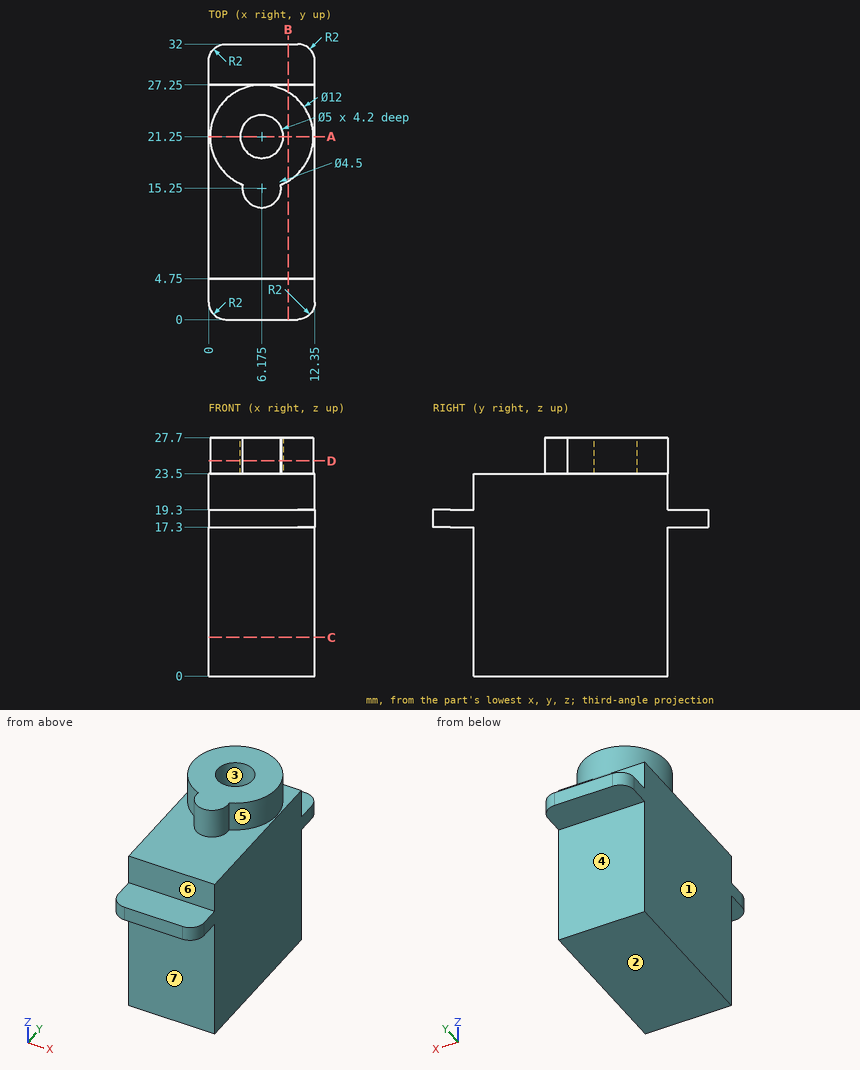
Geometry check sheet. Reference: drawing and pictorial views, mm from the part's lowest x, y, z. A direction names the side the tool comes from. Give positions to 0.01 mm unless a question says otherwise; leave off trailing zeros. Order: outer loops, then holes, each group sorted by start corner. A loop starts at its lowest first (then second) coordinate and runs counter-clockwise, first axis right, second up. Notation, with made-up numbers: (-33, -6.75) - (19, -6.75) arc R15 cw to (19, 13.25) - close; hole circle Ø3 at (44, 47.5). An arc over 180 degrees is marked (long way). Answer as CSV lines item,"result".
1. Section check A-A (y = 21.25). Record the boundary of the cut face in (x, z) (3 decimals).
Result sheet:
outline,"(0, 0) - (12.35, 0) - (12.35, 23.5) - (12.175, 23.5) - (12.175, 27.7) - (8.675, 27.7) - (8.675, 23.5) - (3.675, 23.5) - (3.675, 27.7) - (0.175, 27.7) - (0.175, 23.5) - (0, 23.5) - close"
2. Section check D-D (z = 25). Record the boundary of the cut face in (x, y) (3 decimals), then the cut area to 3 significant figures.
Result sheet:
outline,"(3.965, 15.672) arc R2.25 ccw (long way) to (8.385, 15.672) arc R6 ccw (long way) to start; hole circle Ø5 at (6.175, 21.25)"
area,"102 mm²"
3. Section check C-C (z = 4.5). Record the boundary of the cut face in (x, y), then the cut area to 3 significant figures.
Result sheet:
outline,"(0, 4.75) - (12.35, 4.75) - (12.35, 27.25) - (0, 27.25) - close"
area,"278 mm²"
4. Mould release check, pull along X, two halves, no side actions. Record for the marked faces 1, 2 and 3: released by +X, released by -X, zero draft, split by the parting line, or undercut.
Result sheet:
face 1,"released by -X"
face 2,"zero draft"
face 3,"undercut"
5. Tool access check on the marked faces 4, 5, 6 and 7. Record the directions out of +Z, -Z, +X, -X, +Y, -Y that give a thin tool (end or side, any length) a straight path to the whole face; none if there is none.
Result sheet:
face 4,"-Z, +X, -X, +Y"
face 5,"+Z"
face 6,"+Z, +X, -X, -Y"
face 7,"-Z, +X, -X, -Y"
6. Scan lines: probe 1 along Z at (x, y) = (10.5, 25.5); probe 2 along Y at (x, z) = (2, 15.5); probe 3 along Y at (x, z) = (3.5, 24). Record each from-to range of solid material in increasing order. Write a range as from..to.
Result sheet:
probe 1,"0..23.5"
probe 2,"4.75..27.25"
probe 3,"15.88..26.62"
7. Section check B-B (x = 9.25). Record the boundary of the cut face in (y, z).
Result sheet:
outline,"(0, 17.3) - (4.75, 17.3) - (4.75, 0) - (27.25, 0) - (27.25, 17.3) - (32, 17.3) - (32, 19.3) - (27.25, 19.3) - (27.25, 23.5) - (26.4, 23.5) - (26.4, 27.7) - (16.1, 27.7) - (16.1, 23.5) - (4.75, 23.5) - (4.75, 19.3) - (0, 19.3) - close"
8. Go/stop test with flat-tipped pins: P1, Ø6, axis at x = 5, z = 6, coming from the -Y side; P2, Ø1.5, axis at x = 2, z = 8, coming from the +Y side; P3, Ø4, axis at x = 6.175, y = 21.25, coming from the +Z side. Record where each tip stops, or that it passes through.
Result sheet:
P1,"y = 4.75"
P2,"y = 27.25"
P3,"z = 23.5"
